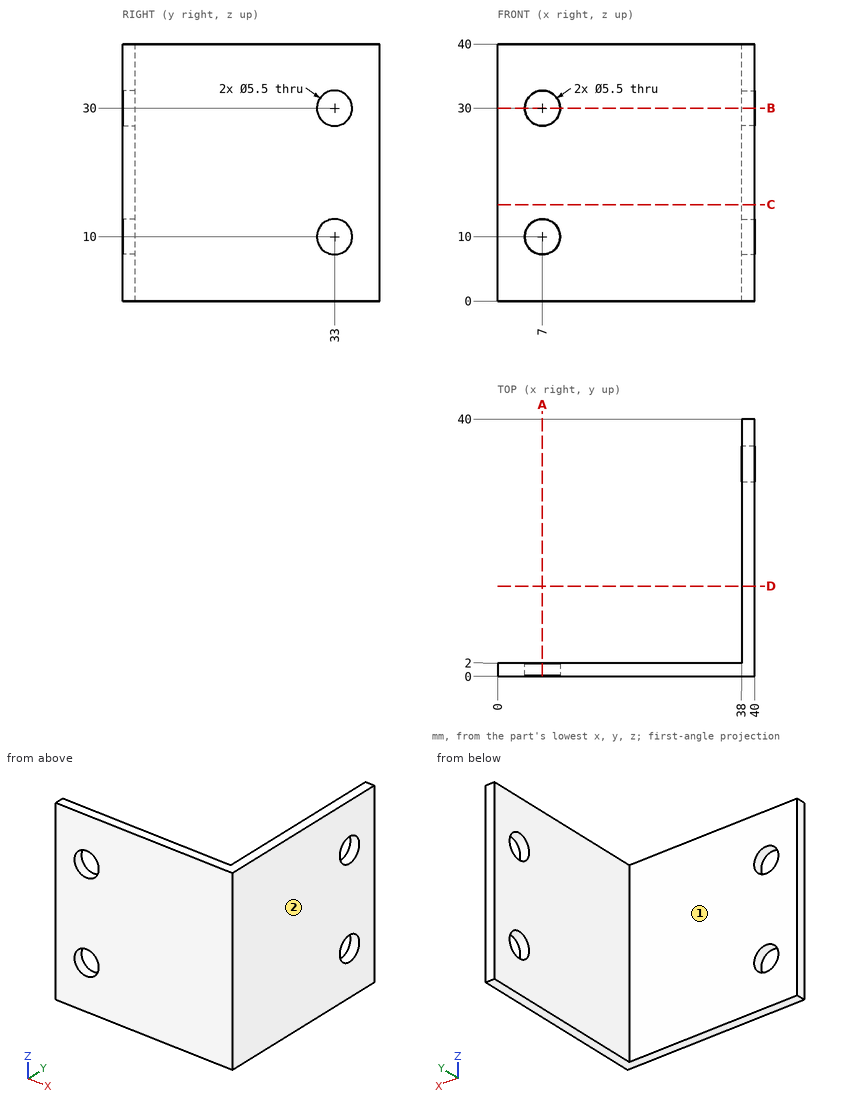
Check sheet for the drawn part. Datum: minimum x, y, z corner. Units: mm. A direction names the side the tool comes from. Coordinates: 2 decimals unless noted, no trailing zeros. Loops run counter-clockwise (first coordinate to the right, second up) from the corner with the lowest first, then second, coordinate; pieces in that order, holes last. Notation, with made-up numbers: (27, -24.5) - (32, -24.5) arc R22 cw to (32, -18.5) - close; hole circle Ø6 at (-15.75, 83.25). An arc over 180 degrees is marked (long way). Put each result on its own line as item: value.
Item 1: Scan lines: line 1 along Z through (x, y) = (7, 1.45); line 2 along X through (y, z) = (0.6, 30); line 3 along Y through (x, z) = (13, 38.5). Record each from-to range of solid material in increasing order.
Conclusion:
line 1: z = 0 to 7.25, 12.75 to 27.25, 32.75 to 40
line 2: x = 0 to 4.25, 9.75 to 40
line 3: y = 0 to 2
Item 2: Gauge pin test, flat ends, axial feed: pin 1 Ø10 at (y, z) = (32, 5) entering from -X; pin 2 Ø9 at (x, z) = (7, 30) entering from +Y. Record the tip position at first contact, or that the pin passes through.
Conclusion:
pin 1: stops at x = 38
pin 2: stops at y = 2
Item 3: Section check D-D (y = 14). Enter the section's corners in (x, z).
Conclusion:
outline: (38, 0) - (40, 0) - (40, 40) - (38, 40) - close
Item 4: Section check B-B (z = 30). Enter the section's corners in (x, y), then the cut area to 3 significant figures.
Conclusion:
outline: (0, 0) - (4.25, 0) - (4.25, 2) - (0, 2) - close; (9.75, 0) - (40, 0) - (40, 30.25) - (38, 30.25) - (38, 2) - (9.75, 2) - close; (38, 35.75) - (40, 35.75) - (40, 40) - (38, 40) - close
area: 134 mm2
Item 5: Section check C-C (z = 15). Enter the section's corners in (x, y), then the cut area to 3 significant figures.
Conclusion:
outline: (0, 0) - (40, 0) - (40, 40) - (38, 40) - (38, 2) - (0, 2) - close
area: 156 mm2
Item 6: Section check A-A (x = 7). Enter the section's corners in (y, z), then the cut area to 3 significant figures.
Conclusion:
outline: (0, 0) - (2, 0) - (2, 7.25) - (0, 7.25) - close; (0, 12.75) - (2, 12.75) - (2, 27.25) - (0, 27.25) - close; (0, 32.75) - (2, 32.75) - (2, 40) - (0, 40) - close
area: 58.0 mm2
Item 7: Set-up check for the marked faces 1 and 2: record each of +Z, -Z, +X, -X, +Y, -Y from which the full face is reachable in a straight line by a thin tool's end or side.
Conclusion:
face 1: +Z, -Z, -X, +Y
face 2: +Z, -Z, +X, +Y, -Y
